from build123d import *

# Parameters (mm, degrees)
SKETCH1_W           = 52
SKETCH1_H           = 26
SKETCH1_R           = 1.7
BOSS_EXTRUDE1_DEPTH = 1
CHAMFER1_SIZE       = 1


with BuildPart() as part:
    # Sketch1 → Boss-Extrude1 (new body)
    with BuildSketch(Plane.XY):
        with Locations((26, -13)):
            Rectangle(SKETCH1_W, SKETCH1_H)
        with Locations((11, -6.344)):
            Circle(SKETCH1_R, mode=Mode.SUBTRACT)
        with Locations((41, -6.344)):
            Circle(SKETCH1_R, mode=Mode.SUBTRACT)
    extrude(amount=BOSS_EXTRUDE1_DEPTH)

    # Chamfer1
    chamfer1_edges = [part.edges().sort_by_distance(p)[0] for p in [
        (0, 0, 0.5),
        (52, 0, 0.5),
        (52, -26, 0.5),
        (0, -26, 0.5),
    ]]
    chamfer(chamfer1_edges, length=CHAMFER1_SIZE)


solid = part.part
Can you work these out from the model? Positions are in its coordinate system, mm. Coordinates: 2 decimals unless noted, no trailing zeros. Write each loop counter-clockwise with the first axis right and the second up, starting at its lowest first coordinate (ties: lowest second). Pieces come first, ordered by that corner, then holes. Notation, with made-up numbers: (-34, 25.25) - (-21, 25.25) arc R18 ccw to (-21, 55.25) - close; hole circle Ø10 at (-2.75, 82.5). An arc over 180 degrees is marked (long way). Return JSON: item names as keys, results as strings. Group by question number.
Item 1: Please list where these lines run through material, in increasing order: probe 1 along X at (y, z) = (-6.5, 0.3); probe 2 along Y at (x, z) = (41, 0.3); probe 3 along Y at (x, z) = (9.5, 0.5).
Item 2: If we section it at B-B (y = -5.5): Write out the boundary of the cut face in (x, z).
Item 3: If we section it at A-A (x = 41): Write out the boundary of the cut face in (y, z).
Item 4: We'd pull the mould along Y, two halves only. Please class faces 1 (the face through (26, -13, 1)), 2 (the face through (0.5, -25.5, 0.5)), 3 (the face through (51.5, -0.5, 0.5)), 4 (the face through (39.65, -7.38, 0.49)): pulls with the +Y half, pulls with the -Y half, needs draft (parallel to the pull), parting line crosses it, or undercut.
Return value:
{
 "1": {"probe 1": "x = 0 to 9.31, 12.69 to 39.31, 42.69 to 52", "probe 2": "y = -26 to -8.04, -4.64 to 0", "probe 3": "y = -26 to -7.14, -5.54 to 0"},
 "2": {"outline": "(0, 0) - (9.52, 0) - (9.52, 1) - (0, 1) - close; (12.48, 0) - (39.52, 0) - (39.52, 1) - (12.48, 1) - close; (42.48, 0) - (52, 0) - (52, 1) - (42.48, 1) - close"},
 "3": {"outline": "(-26, 0) - (-8.04, 0) - (-8.04, 1) - (-26, 1) - close; (-4.64, 0) - (0, 0) - (0, 1) - (-4.64, 1) - close"},
 "4": {"face 1": "needs draft", "face 2": "pulls with the -Y half", "face 3": "pulls with the +Y half", "face 4": "undercut"}
}
